from build123d import *

# Parameters (mm, degrees)
F0_W     = 57.15
F0_H     = 38.1
F1_DEPTH = 25.4
F3_DEPTH = 25.4
F5_DEPTH = 25.4


with BuildPart() as f1:
    # F0 (on Front) → F1 (new body)
    with BuildSketch(Plane.XZ):
        with Locations((-7.0866, 19.05)):
            Rectangle(F0_W, F0_H)
    extrude(amount=F1_DEPTH)

    # F2 (on face) → F3 (cut)
    with BuildSketch(Plane.XZ.offset(25.4)):
        with BuildLine():
            Line((21.4884, 38.1), (2.4384, 38.1))
            ThreePointArc((2.4384, 38.1), (8.018016, 24.629616), (21.4884, 19.05))
            Line((21.4884, 19.05), (21.4884, 38.1))
        make_face()
    extrude(amount=-F3_DEPTH, mode=Mode.SUBTRACT)

    # F4 (on face) → F5 (cut)
    with BuildSketch(Plane.XZ.offset(25.4)):
        with BuildLine():
            ThreePointArc((-35.6616, 31.75), (-33.772823, 36.211223), (-29.3116, 38.1))
            Line((-29.3116, 38.1), (-35.6616, 38.1))
            Line((-35.6616, 38.1), (-35.6616, 31.75))
        make_face()
    extrude(amount=-F5_DEPTH, mode=Mode.SUBTRACT)


solid = f1.part
Read the model definition and answer for the solid it produces. Units are mm, in the model's axes. Round coordinates to 2 decimals unless told otherwise and drop trailing zeros. Loops run counter-clockwise (first coordinate to the right, second up) from the corner with the lowest first, then second, coordinate; pieces in that order, holes last.
Q1. Determine the mould class of faces 1 (the face through (-35.662, -13, 16)), 2 (the face through (21.488, -13, 9)), 3 (the face through (-7, -13, 0)) for opening direction X: released by +X, released by -X, zero draft, split by the parting line, or undercut.
Q2. This flat-tipped pin is pushed along its axis until it touches: pin 1 (4 mm diameter, centred on y = -18.5, z = 29, fed in from +X). Where does it stop, or does it pass through?
Q3. Section B-B on z = 33.5 is taken. Write down the section's boundary in (x, y).
Q4. Section C-C on x = 13 is taken. Write down the section's boundary in (y, z), and give its area (3 significant figures).
Q5. Consider probe 1 along Z at (x, y) = (-29.5, -15.75); probe 2 along X at (y, z) = (-17, 36); probe 3 along Z at (x, y) = (9, -17). Determine where each line is inside the solid, lowest interval first.
Q6. Section A-A on y = -18 is taken. Write down the section's boundary in (x, z).
Output:
1. face 1: released by -X
1. face 2: released by +X
1. face 3: zero draft
2. pin 1: stops at x = 6.01
3. outline: (-35.39, -25.4) - (3, -25.4) - (3, 0) - (-35.39, 0) - close
4. outline: (-25.4, 0) - (0, 0) - (0, 21.05) - (-25.4, 21.05) - close
4. area: 535 mm2
5. probe 1: z = 0 to 38.09
5. probe 2: x = -33.97 to 2.55
5. probe 3: z = 0 to 23.71
6. outline: (-35.66, 0) - (21.49, 0) - (21.49, 19.05) arc R19.05 cw to (2.44, 38.1) - (-29.31, 38.1) arc R6.45 ccw to (-35.66, 31.75) - close
